from build123d import *

# Parameters (mm, degrees)
BOSS_EXTRUDE1_DEPTH = 4


with BuildPart() as part:
    # Sketch2 → Boss-Extrude1 (new body)
    with BuildSketch(Plane.XY):
        with BuildLine():
            Line((262.480297025, 7.13882444), (262.480297025, -7.13882444))
            add(Edge.make_bspline(
                [(211.080761054, -14.13724363), (211.917848379, -13.89687615), (219.460294723, -11.745335639), (236.298901932, -7.327257032), (252.970465499, -6.414227327), (262.480297025, -7.13882444)],
                knots=[0.460880267, 0.460880267, 0.460880267, 0.460880267, 0.487879211, 0.704009033, 1, 1, 1, 1], degree=3))
            Line((211.080761054, -14.13724363), (211.080761054, -9.13724363))
            Line((211.080761054, -9.13724363), (142.548046426, -9.13724363))
            Line((142.548046426, -9.13724363), (142.548046426, 9.13724363))
            Line((142.548046426, 9.13724363), (211.080761054, 9.13724363))
            Line((211.080761054, 9.13724363), (211.080761054, 14.13724363))
            add(Edge.make_bspline(
                [(211.080761054, 14.13724363), (211.917848379, 13.89687615), (219.460294722, 11.745335639), (236.298901932, 7.327257032), (252.970465499, 6.414227327), (262.480297025, 7.13882444)],
                knots=[0.460880267, 0.460880267, 0.460880267, 0.460880267, 0.487879211, 0.704009033, 1, 1, 1, 1], degree=3))
        make_face()
    extrude(amount=BOSS_EXTRUDE1_DEPTH)


solid = part.part
Geometry check sheet. Reference: the model listing, model coordinates, mm. A direction names the side the tool comes from. Give positions to 0.01 mm unless a question says otherwise; leave off trailing zeros. Write each loop counter-clockwise with the first axis right and the second up, starting at its lowest first coordinate (ties: lowest second). Pieces come first, ordered by that corner, then holes.
1) Thickness scan on line 1 (Y direction, x = 167.5, z = 3.75); line 2 (Y direction, x = 250, z = 0.7). Record the ranges inside material, lowest first.
Values follow:
line 1: y = -9.14 to 9.14
line 2: y = -6.89 to 6.89
2) Set-up check for faces 1 (the face through (203, 0, 4)), 2 (the face through (176, 9.137, 2)), 3 (the face through (211.081, -12, 2)): record each of +Z, -Z, +X, -X, +Y, -Y from which the full face is reachable in a straight line by a thin tool's end or side.
Values follow:
face 1: +Z, +X, -X, +Y, -Y
face 2: +Z, -Z, -X, +Y
face 3: +Z, -Z, -X, -Y
3) Go/stop test with flat-tipped pins: pin 1 Ø1.5 at (x, z) = (178.5, 3) entering from -Y; pin 2 Ø2 at (x, z) = (190.5, 1.5) entering from +Y. Record where each tip stops, or that it passes through.
Values follow:
pin 1: stops at y = -9.14
pin 2: stops at y = 9.14
4) Cross-section at A-A (x = 185). Record the boundary of the cut face in (y, z), plus the area to 3 significant figures.
Values follow:
outline: (-9.14, 0) - (9.14, 0) - (9.14, 4) - (-9.14, 4) - close
area: 73.1 mm2
